Model file for the job. Use its own axes, mm. Face numbers are marked on the shaded views. A direction names the side the tool comes from. Round coordinates to 2 decimals unless told otherwise and drop trailing zeros. Write each loop counter-clockwise with the first axis right and the second up, starting at its lowest first coordinate (ties: lowest second). Pieces come first, ordered by that corner, then holes. Notation, with made-up numbers: (-22.75, 47) - (22.25, 47) arc R30 cw to (22.25, 84) - close; hole circle Ø3 at (-9.5, -21.75). An arc over 180 degrees is marked (long way). One line per item, written item: value.
from build123d import *

# Parameters (mm, degrees)
SKETCH1_W           = 50
SKETCH1_H           = 47.7
SKETCH1_R           = 1.75
SKETCH1_R_2         = 3.81
BOSS_EXTRUDE1_DEPTH = 3.175
SKETCH2_W           = 50
SKETCH2_H           = 3.175
BOSS_EXTRUDE2_DEPTH = 30.5976
SKETCH3_W           = 50
SKETCH3_H           = 3.175
BOSS_EXTRUDE3_DEPTH = 15
CUT_EXTRUDE1_REACH  = 62.585
SKETCH4_R           = 1.7859375


with BuildPart() as part:
    # Sketch1 → Boss-Extrude1 (new body)
    with BuildSketch(Plane.XY):
        with Locations((-10, 0)):
            Rectangle(SKETCH1_W, SKETCH1_H)
        with Locations((-24, 9)):
            Circle(SKETCH1_R, mode=Mode.SUBTRACT)
        with Locations((-24, -9)):
            Circle(SKETCH1_R, mode=Mode.SUBTRACT)
        with Locations((9, -9)):
            Circle(SKETCH1_R, mode=Mode.SUBTRACT)
        with Locations((9, 9)):
            Circle(SKETCH1_R, mode=Mode.SUBTRACT)
        Circle(SKETCH1_R_2, mode=Mode.SUBTRACT)
    extrude(amount=BOSS_EXTRUDE1_DEPTH)

    # Sketch2 → Boss-Extrude2 (add)
    with BuildSketch(Plane(origin=(0, 0, 0), x_dir=(-1, 0, 0), z_dir=(0, 0, -1))):
        with Locations((10, -22.2625)):
            Rectangle(SKETCH2_W, SKETCH2_H)
        with Locations((10, 22.2625)):
            Rectangle(SKETCH2_W, SKETCH2_H)
    extrude(amount=BOSS_EXTRUDE2_DEPTH)

    # Sketch3 → Boss-Extrude3 (add)
    with BuildSketch(Plane(origin=(0, 23.85, 0), x_dir=(1, 0, 0), z_dir=(0, 1, 0))):
        with Locations((-10, 29.0101)):
            Rectangle(SKETCH3_W, SKETCH3_H)
    boss_extrude3 = extrude(amount=BOSS_EXTRUDE3_DEPTH)

    # Sketch4 → Cut-Extrude1 (cut, up to next)
    with BuildSketch(Plane.XY.offset(-27.4226), mode=Mode.PRIVATE) as cut_extrude1_sk1:
        with Locations((2.7, 31.35)):
            Circle(SKETCH4_R)
    cut_extrude1_tool1 = extrude(cut_extrude1_sk1.sketch, amount=-CUT_EXTRUDE1_REACH, mode=Mode.PRIVATE) & part.part
    # Sketch4 → Cut-Extrude1 (cut, up to next)
    with BuildSketch(Plane.XY.offset(-27.4226), mode=Mode.PRIVATE) as cut_extrude1_sk2:
        with Locations((-22.7, 31.35)):
            Circle(SKETCH4_R)
    cut_extrude1_tool2 = extrude(cut_extrude1_sk2.sketch, amount=-CUT_EXTRUDE1_REACH, mode=Mode.PRIVATE) & part.part
    cut_extrude1_1 = cut_extrude1_tool1.solids().sort_by_distance((2.7, 31.35, -27.4226))[0]
    add(cut_extrude1_1, mode=Mode.SUBTRACT)
    cut_extrude1_2 = cut_extrude1_tool2.solids().sort_by_distance((-22.7, 31.35, -27.4226))[0]
    add(cut_extrude1_2, mode=Mode.SUBTRACT)
    cut_extrude1 = cut_extrude1_1 + cut_extrude1_2  # Cut-Extrude1 as one shape, for the pattern or mirror that repeats it

    # Mirror1: Boss-Extrude3, Cut-Extrude1 across plane
    add(boss_extrude3.mirror(Plane.ZX))
    add(cut_extrude1.mirror(Plane.ZX), mode=Mode.SUBTRACT)


solid = part.part
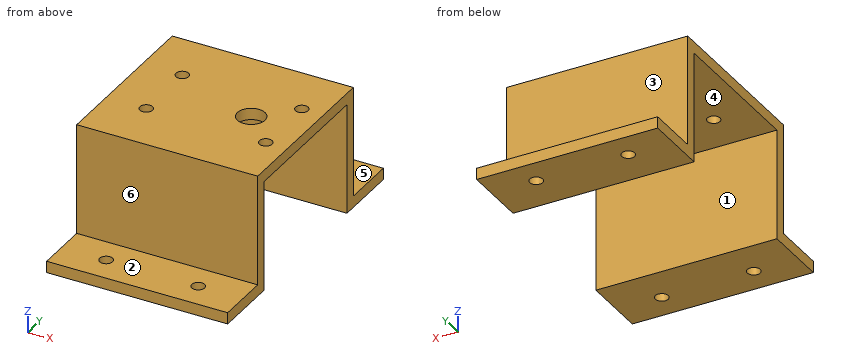
1. Band-saw the part on C-C on x = 9. Write the cut outline in (y, z) (3 decimals), plus the area to 3 significant figures.
Report:
outline: (-38.85, -30.598) - (-20.675, -30.598) - (-20.675, 0) - (-10.75, 0) - (-10.75, 3.175) - (-23.85, 3.175) - (-23.85, -27.423) - (-38.85, -27.423) - close; (-7.25, 0) - (7.25, 0) - (7.25, 3.175) - (-7.25, 3.175) - close; (10.75, 0) - (20.675, 0) - (20.675, -30.598) - (38.85, -30.598) - (38.85, -27.423) - (23.85, -27.423) - (23.85, 3.175) - (10.75, 3.175) - close
area: 419 mm²
2. Band-saw the part on B-B on y = 9. Write the cut outline in (x, z) (3 decimals), plus the area to 3 significant figures.
Report:
outline: (-35, 0) - (-25.75, 0) - (-25.75, 3.175) - (-35, 3.175) - close; (-22.25, 0) - (7.25, 0) - (7.25, 3.175) - (-22.25, 3.175) - close; (10.75, 0) - (15, 0) - (15, 3.175) - (10.75, 3.175) - close
area: 137 mm²
3. Drop flat-ended pins along their axis: pin 1 (5 mm diameter, centred on x = -21, z = -3.5, fed in from +Y); pin 2 (3 mm diameter, centred on x = -22.7, y = 31.35, fed in from -Z); pin 3 (7.5 mm diameter, centred on x = -11.5, y = -32, fed in from +Z); pin 4 (10 mm diameter, centred on x = -5.5, y = -7.5, fed in from -Z). Give the stop position or say it passes through.
Report:
pin 1: y = 23.85
pin 2: through
pin 3: z = -27.42
pin 4: z = 0
4. Mould opens along Y. For the marked faces 1, 2 and 3 say: released by +Y, released by -Y, zero draft, split by the parting line, or undercut.
Report:
face 1: undercut
face 2: zero draft
face 3: released by +Y
5. Tool access for the marked faces 4, 5 and 6: list every direction of +Z, -Z, +X, -X, +Y, -Y with a clear straight run to the whole face (end or side of a thin tool).
Report:
face 4: -Z, +X, -X
face 5: +Z, +X, -X, +Y
face 6: +Z, +X, -X, -Y
6. Wall check: probe 1 along Y at (x, z) = (-24, 1); probe 2 along X at (y, z) = (-31.35, -28.95); probe 3 along Y at (x, z) = (-3.5, -27) (3 decimals). Give the ranges that are in metal, low to high. Write a range as [from, to].
Report:
probe 1: [-23.85, -10.75], [-7.25, 7.25], [10.75, 23.85]
probe 2: [-35, -24.49], [-20.91, 0.91], [4.49, 15]
probe 3: [-23.85, -20.675], [20.675, 23.85]
7. Band-saw the part on A-A on z = -14. Write the cut outline in (x, y) (3 decimals), plus the area to 4 significant figures.
Report:
outline: (-35, -23.85) - (15, -23.85) - (15, -20.675) - (-35, -20.675) - close; (-35, 20.675) - (15, 20.675) - (15, 23.85) - (-35, 23.85) - close
area: 317.5 mm²
8. Band-saw the part on D-D on x = -30. Write the cut outline in (y, z) (3 decimals).
Report:
outline: (-38.85, -30.598) - (-20.675, -30.598) - (-20.675, 0) - (20.675, 0) - (20.675, -30.598) - (38.85, -30.598) - (38.85, -27.423) - (23.85, -27.423) - (23.85, 3.175) - (-23.85, 3.175) - (-23.85, -27.423) - (-38.85, -27.423) - close
